Design review of the part shown in the three views and the two pictorial views. Dimensions are in mm from the part's minimum x, y and z. A direction names the side the tool comes from. Give positions to 0.01 mm unless a question says otherwise; leave off trailing zeros. Order: outer loops, then holes, each group sorted by start corner. A loop starts at its lowest first (then second) coordinate and runs counter-clockwise, first axis right, second up.
Item 1: Consider section D-D (z = 10.5). Give the boundary of the cut face in (x, y), plus the area to 3 significant figures.
Item 2: Machinability: for the marked faces 5 and 6, which of the approach directions +Z, -Z, +X, -X, +Y, -Y give a long, thin tool a straight path to every point of the face, cutting with its end or side? Answer none if there is none.
Item 3: Consider section A-A (y = 16). Give the boundary of the cut face in (x, z), plus the area to 3 significant figures.
Item 4: For probe 1 along X at (y, z) = (13.5, 3); probe 2 along Y at (x, z) = (17.5, 20); probe 3 along Y at (x, z) = (8, 37), list the stretches that pass through material, from the lowest coordinate up.
Item 5: For P1, Ø1, axis at x = 43, z = 26.5, coming from the -Y side; P2, Ø24, axis at x = 25.5, z = 14.5, coming from the +Y side, all flat-tipped, find the tip position at first contact; note any pin that passes through.
Item 6: The part is to be moulded in two halves that separate along X. For the marked faces 1, 2, 3 and 4, say which applies: released by +X, released by -X, zero draft, split by the parting line, or undercut.
Item 7: Consider section C-C (x = 42). Give the boundary of the cut face in (y, z) (1 decimal), plus the area to 3 significant figures.
Item 8: Consider section B-B (z = 16). Give the boundary of the cut face in (x, y), plus the area to 3 significant figures.
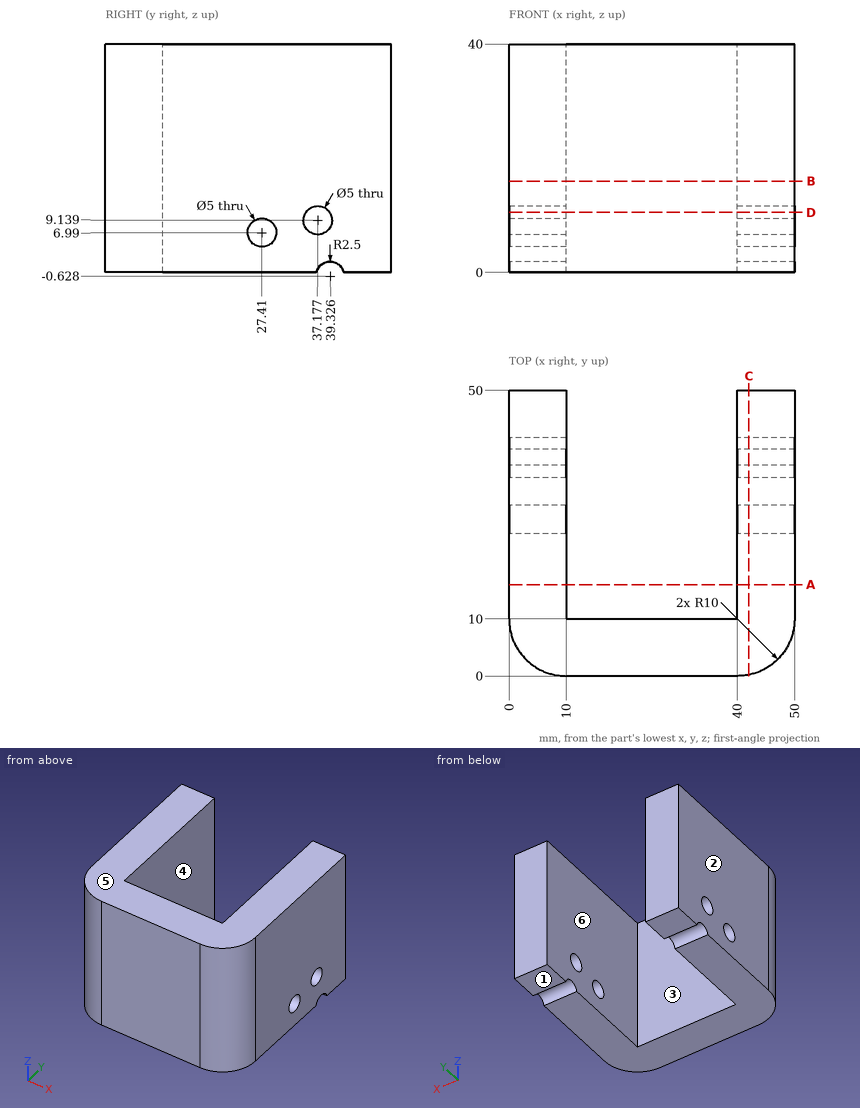
Resolved:
1. outline: (0, 10) arc R10 ccw to (10, 0) - (40, 0) arc R10 ccw to (50, 10) - (50, 35.08) - (40, 35.08) - (40, 10) - (10, 10) - (10, 35.08) - (0, 35.08) - close; (0, 39.27) - (10, 39.27) - (10, 50) - (0, 50) - close; (40, 39.27) - (50, 39.27) - (50, 50) - (40, 50) - close
1. area: 1,170 mm2
2. face 5: +Z, +X, -X, +Y, -Y
2. face 6: +Z, -Z, +Y
3. outline: (0, 0) - (10, 0) - (10, 40) - (0, 40) - close; (40, 0) - (50, 0) - (50, 40) - (40, 40) - close
3. area: 800 mm2
4. probe 1: x = 0 to 10, 40 to 50
4. probe 2: y = 0 to 10
4. probe 3: y = 0.2 to 50
5. P1: stops at y = 0.32
5. P2: stops at y = 10
6. face 1: zero draft
6. face 2: released by -X
6. face 3: undercut
6. face 4: undercut
7. outline: (0.2, 0) - (36.9, 0) arc R2.5 cw to (41.7, 0) - (50, 0) - (50, 40) - (0.2, 40) - close; hole circle Ø5 at (27.4, 7); hole circle Ø5 at (37.2, 9.1)
7. area: 1,950 mm2
8. outline: (0, 10) arc R10 ccw to (10, 0) - (40, 0) arc R10 ccw to (50, 10) - (50, 50) - (40, 50) - (40, 10) - (10, 10) - (10, 50) - (0, 50) - close
8. area: 1,260 mm2
